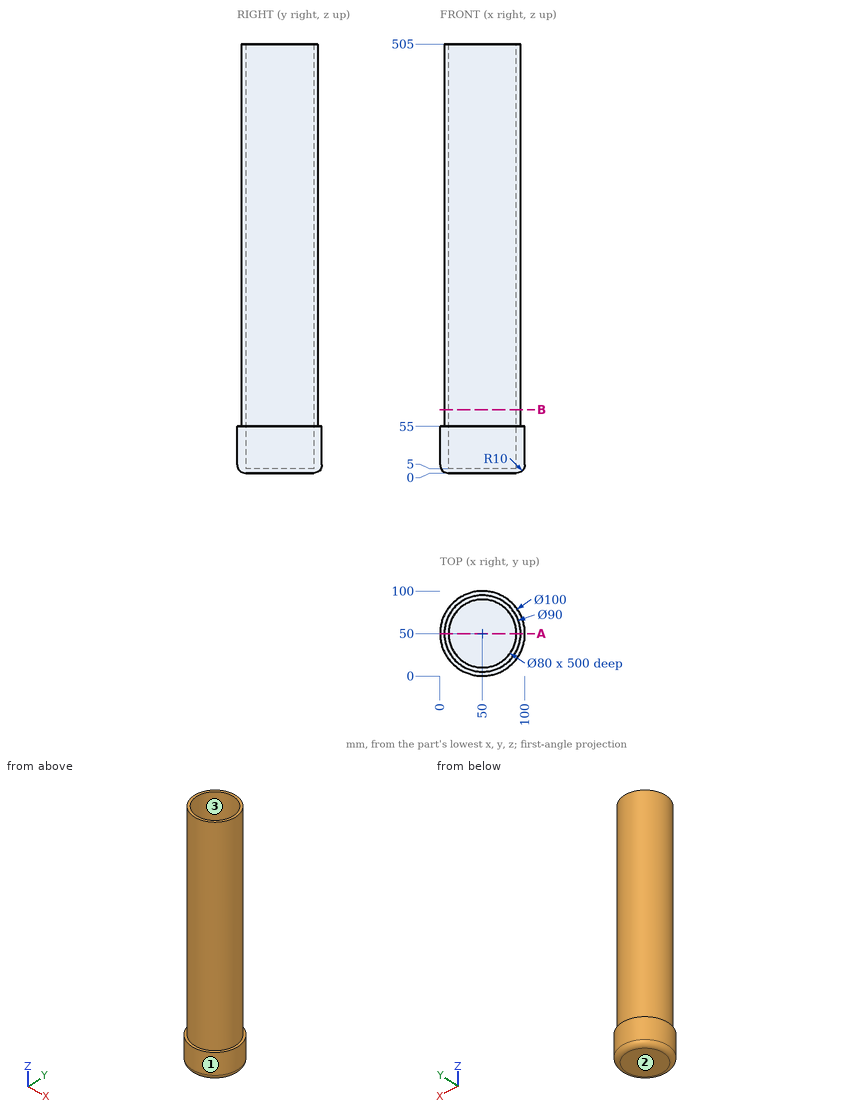
Study the drawing (mm; zero at the part's minimum x, y, z) and answer. Give positions to 0.01 mm unless a question says otherwise; leave off trailing zeros. Order: outer loops, then holes, each group sorted by start corner. A loop starts at its lowest first (then second) coordinate and runs counter-clockwise, first axis right, second up.
1. Each of these flat-tipped pins is pushed along its axis until it touches: P1, Ø2, axis at y = 89, z = 233, coming from the +X side; P2, Ø3, axis at y = 62, z = 201.5, coming from the -X side; P3, Ø1, axis at y = 72.5, z = 157, coming from the -X side. Where does it stop, or does it pass through?
Result sheet:
P1: stops at x = 74.1
P2: stops at x = 6.24
P3: stops at x = 10.74
2. The mould has two halves that part along X. Classify the marked faces 1, 2 and 3: released by +X, released by -X, zero draft, split by the parting line, or undercut.
Result sheet:
face 1: split by the parting line
face 2: zero draft
face 3: undercut
3. Section A-A, the plane y = 50 is taken. Determine the outline of the cut face in (x, z), and give its area (3 significant figures).
Result sheet:
outline: (0, 10) arc R10 ccw to (10, 0) - (90, 0) arc R10 ccw to (100, 10) - (100, 55) - (95, 55) - (95, 505) - (90, 505) - (90, 5) - (10, 5) - (10, 505) - (5, 505) - (5, 55) - (0, 55) - close
area: 5,960 mm2
4. Straight lines are drawn through the part: L1, parallel to Y at x = 51, z = 314.5; L2, parallel to Z at x = 59.5, y = 56.5; L3, parallel to X at y = 70, z = 36. For each, find the intervals that lie inside material, in ascending order.
Result sheet:
L1: y = 5.01 to 10.01, 89.99 to 94.99
L2: z = 0 to 5
L3: x = 4.17 to 15.36, 84.64 to 95.83
5. Section B-B, the plane z = 74.5 is taken. Determine the outline of the cut face in (x, y).
Result sheet:
outline: circle Ø90 at (50, 50); hole circle Ø80 at (50, 50)
